Autodesk Inventor part; units mm, degrees
ref_plane "YZ Plane" through (0, 0, 0) normal (1, 0, 0) x (0, 1, 0)
ref_plane "XZ Plane" through (0, 0, 0) normal (0, 1, 0) x (-1, 0, 0)
ref_plane "XY Plane" through (0, 0, 0) normal (0, 0, 1) x (1, 0, 0)
sketch "Sketch1" plane through (0, 0, 0) normal (0, 0, 1) x (1, 0, 0)
  line L0 (-6.35, -3.6662) -> (-6.35, 3.6662)
  line L1 (-6.35, 3.6662) -> (0, 7.3323)
  line L2 (0, 7.3323) -> (6.35, 3.6662)
  line L3 (6.35, 3.6662) -> (6.35, -3.6662)
  line L4 (6.35, -3.6662) -> (0, -7.3323)
  line L5 (0, -7.3323) -> (-6.35, -3.6662)
  point P0 (0, 0)
  point P1 (0, 0)
  dimension "Size" = 12.7
extrude "Extrusion1" add sketch "Sketch1" along normal mid plane 14.6114
sketch "Sketch2" plane through (0, 0, 7.3057) normal (0, 0, 1) x (1, 0, 0)
  line L0 (-6.35, 3.6662) -> (-6.35, -3.6662) construction
  line L1 (-6.35, -3.6662) -> (0, -7.3323) construction
  line L2 (0, -7.3323) -> (6.35, -3.6662) construction
  line L3 (6.35, -3.6662) -> (6.35, 3.6662) construction
  line L4 (6.35, 3.6662) -> (0, 7.3323) construction
  line L5 (0, 7.3323) -> (-6.35, 3.6662) construction
  circle A0 centre (0, 0) radius 6.35
extrude "Extrusion2" add sketch "Sketch2" along normal blind 7.9248
mirror "Mirror1" about plane through (0, 0, 0) normal (0, 0, 1) of "Extrusion2"
properties part number "EL2-CGB-011" material "Aluminum 6061"
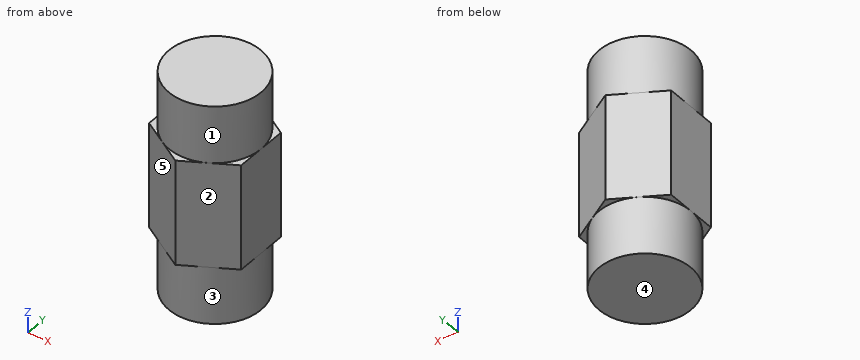
Geometry check sheet. Reference: the model listing, model coordinates, mm. Face numbers are marked on the shaded views. A direction names the side the tool comes from. Round coordinates to 2 decimals unless told otherwise and drop trailing zeros. Write each loop counter-clockwise with the first axis right and the second up, starting at its lowest first coordinate (ties: lowest second). Pieces come first, ordered by that corner, then holes. Notation, with made-up numbers: (54.25, 67.5) - (82.25, 67.5) arc R16 cw to (82.25, 76.5) - close; hole circle Ø8 at (16.5, 62.25). An arc over 180 degrees is marked (long way). One line per item, written item: value.
1. Cross-section at A-A on z = 3.5. Record the boundary of the cut face in (x, y), and give its area (3 significant figures).
The answers:
outline: (-6.35, -3.67) - (0, -7.33) - (6.35, -3.67) - (6.35, 3.67) - (0, 7.33) - (-6.35, 3.67) - close
area: 140 mm^2
2. Depth check by flat-ended pin: pin 1 Ø1 at (x, z) = (5, 12) entering from +Y; pin 2 Ø3 at (x, z) = (4, -3) entering from +Y; pin 3 Ø6 at (x, z) = (-2, 0.5) entering from +Y. Enter the tip coordinate at first touch or a pass-through.
The answers:
pin 1: stops at y = 4.48
pin 2: stops at y = 5.89
pin 3: stops at y = 7.33
3. Scan lines: L1, parallel to Y at x = 2.75, z = -8; L2, parallel to X at y = 3.75, z = -4; L3, parallel to Y at x = -1, z = 10.5. Record each from-to range of solid material in increasing order.
The answers:
L1: y = -5.72 to 5.72
L2: x = -6.2 to 6.2
L3: y = -6.27 to 6.27
4. Set-up check for the marked faces 1 and 2: record each of +Z, -Z, +X, -X, +Y, -Y from which the full face is reachable in a straight line by a thin tool's end or side.
The answers:
face 1: +Z
face 2: +Z, -Z, +X, -Y
5. Mould release check, pull along X, two halves, no side actions. Record for the marked faces 3, 4 and 5: released by +X, released by -X, zero draft, split by the parting line, or undercut.
The answers:
face 3: split by the parting line
face 4: zero draft
face 5: released by -X
6. Cross-section at B-B on x = 4. Record the boundary of the cut face in (y, z).
The answers:
outline: (-5.02, -7.31) - (-4.93, -7.31) - (-4.93, -15.23) - (4.93, -15.23) - (4.93, -7.31) - (5.02, -7.31) - (5.02, 7.31) - (4.93, 7.31) - (4.93, 15.23) - (-4.93, 15.23) - (-4.93, 7.31) - (-5.02, 7.31) - close
7. Cross-section at C-C on y = 2. Record the boundary of the cut face in (x, z), and give its area (3 significant figures).
The answers:
outline: (-6.35, -7.31) - (-6.03, -7.31) - (-6.03, -15.23) - (6.03, -15.23) - (6.03, -7.31) - (6.35, -7.31) - (6.35, 7.31) - (6.03, 7.31) - (6.03, 15.23) - (-6.03, 15.23) - (-6.03, 7.31) - (-6.35, 7.31) - close
area: 377 mm^2
